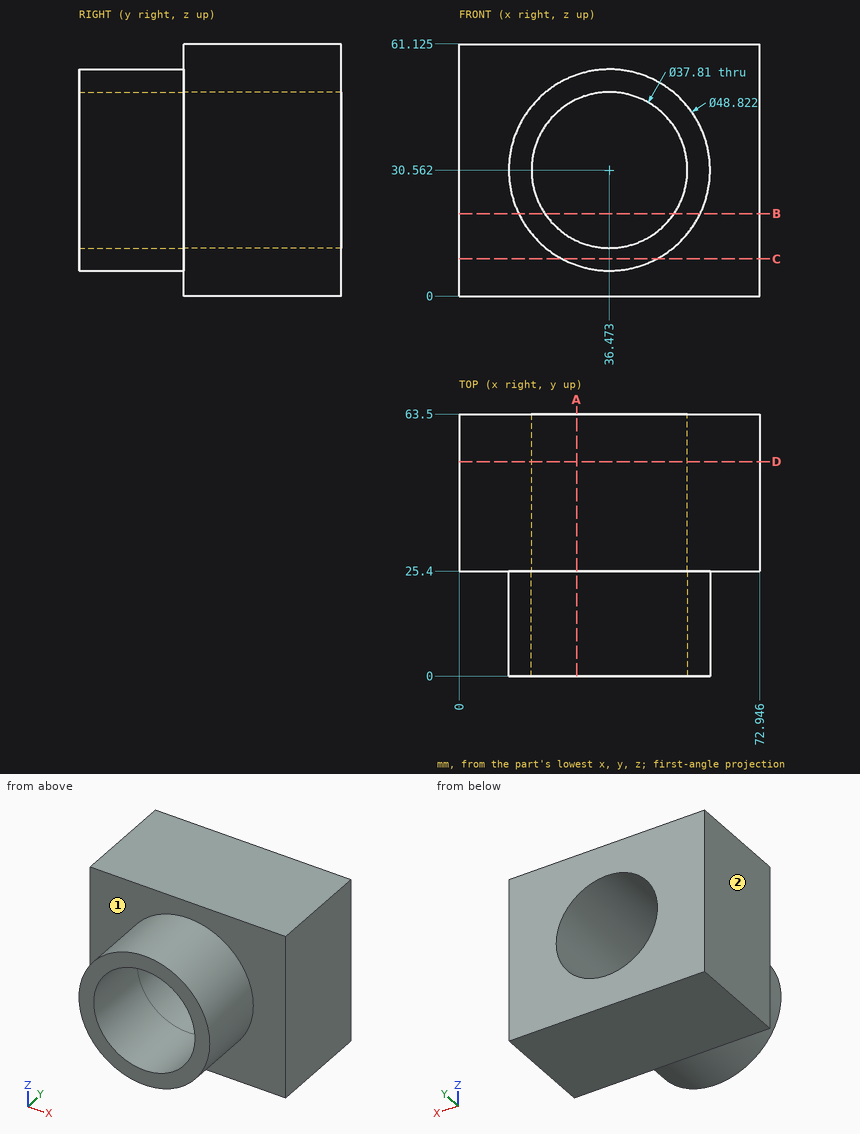
Study the drawing (mm; zero at the part's minimum x, y, z) and answer. A direction names the side the tool comes from. Coordinates: 2 decimals unless noted, no trailing zeros. Write each loop counter-clockwise with the first axis right and the second up, starting at its lowest first coordinate (ties: lowest second). Pieces come first, ordered by that corner, then holes. Notation, with made-up numbers: (34, 20.5) - (52, 20.5) arc R13 cw to (52, 29.5) - close; hole circle Ø10 at (5, 54). An arc over 180 degrees is marked (long way). One line per question, with ' | ' between items.
1) Consider probe 1 along Y at (x, z) = (22, 8); probe 2 along X at (y, z) = (49, 25) (1 decimal); probe 3 along X at (y, z) = (39, 29.5). Determine where each line is inside the solid, lowest interval first. Write a range as [from, to].
Checks:
probe 1: [25.4, 63.5] | probe 2: [0, 18.4], [54.5, 72.9] | probe 3: [0, 17.6], [55.35, 72.95]
2) For the marked faces 1 and 2, determine the directions among +Z, -Z, +X, -X, +Y, -Y from which every point of the face is accessible in a straight line to the end or side of a thin tool.
Checks:
face 1: -Y | face 2: +Z, -Z, -X, +Y, -Y
3) Find section D-D, the plane y = 52. Determine the outline of the cut face in (x, z) (1 decimal), and give its area (3 significant figures).
Checks:
outline: (0, 0) - (72.9, 0) - (72.9, 61.1) - (0, 61.1) - close; hole circle Ø37.8 at (36.5, 30.6) | area: 3,340 mm2
4) Find section C-C, the plane z = 9. Determine the outline of the cut face in (x, y), and give its area (3 significant figures).
Checks:
outline: (0, 25.4) - (25.03, 25.4) - (25.03, 0) - (47.92, 0) - (47.92, 25.4) - (72.95, 25.4) - (72.95, 63.5) - (0, 63.5) - close | area: 3,360 mm2
5) Find section A-A, the plane x = 28.5. Determine the outline of the cut face in (y, z) (1 decimal).
Checks:
outline: (0, 7.5) - (25.4, 7.5) - (25.4, 0) - (63.5, 0) - (63.5, 13.4) - (0, 13.4) - close; (0, 47.7) - (63.5, 47.7) - (63.5, 61.1) - (25.4, 61.1) - (25.4, 53.6) - (0, 53.6) - close
6) Flat-ended cylindrical pins translate along their axes: P1, Ø5, axis at y = 42.5, z = 19.5, coming from the -X side; P2, Ø1, axis at x = 31.5, y = 22.5, coming from the -Z side (1 decimal). Find the tip coordinate at first contact, or state that the pin passes through.
Checks:
P1: x = 0 | P2: z = 6.6
7) Find section B-B, the plane z = 20. Determine the outline of the cut face in (x, y) (1 decimal).
Checks:
outline: (0, 25.4) - (14.5, 25.4) - (14.5, 0) - (20.8, 0) - (20.8, 63.5) - (0, 63.5) - close; (52.2, 0) - (58.5, 0) - (58.5, 25.4) - (72.9, 25.4) - (72.9, 63.5) - (52.2, 63.5) - close
